from build123d import *

# Parameters (mm, degrees)
F0_R          = 2.5
F1_DEPTH      = 1.5
F1_DEPTH_BACK = 1.5
F3_DEPTH      = 2
F2_R          = 5.7
F2_R_2        = 4.2
F4_DEPTH      = 10


with BuildPart() as f1:
    # F0 (on Right) → F1 (new body, two sides)
    with BuildSketch(Plane.YZ) as f1_sk:
        with BuildLine():
            ThreePointArc((-5.5, 0), (0, -5.5), (5.5, 0))
            ThreePointArc((5.5, 0), (0, 5.5), (-5.5, 0))
        make_face()
        Circle(F0_R, mode=Mode.SUBTRACT)
        with BuildLine():
            Line((5.5, -6), (5.5, 0))
            ThreePointArc((5.5, 0), (0, -5.5), (-5.5, 0))
            Line((-5.5, 0), (-5.5, -6))
            Line((-5.5, -6), (5.5, -6))
        make_face()
    extrude(amount=F1_DEPTH)
    extrude(f1_sk.sketch, amount=-F1_DEPTH_BACK)

    # F2 (on face) → F3 (join)
    with BuildSketch(Plane(origin=(0, 0, -6), x_dir=(1, 0, 0), z_dir=(0, 0, -1))):
        with BuildLine():
            ThreePointArc((1.5, -3.9230090492), (3.4597687784, -2.38117618), (4.2, 0))
            ThreePointArc((4.2, 0), (3.4597687784, 2.38117618), (1.5, 3.9230090492))
            Line((1.5, 3.9230090492), (1.5, -3.9230090492))
        make_face()
        with BuildLine():
            Line((1.5, -3.9230090492), (1.5, 3.9230090492))
            ThreePointArc((1.5, 3.9230090492), (0, 4.2), (-1.5, 3.9230090492))
            Line((-1.5, 3.9230090492), (-1.5, -3.9230090492))
            ThreePointArc((-1.5, -3.9230090492), (0, -4.2), (1.5, -3.9230090492))
        make_face()
        with BuildLine():
            Line((-1.5, -3.9230090492), (-1.5, 3.9230090492))
            ThreePointArc((-1.5, 3.9230090492), (-4.2, 0), (-1.5, -3.9230090492))
        make_face()
    extrude(amount=F3_DEPTH)

    # F2 (on face) → F4 (join)
    with BuildSketch(Plane(origin=(0, 0, -6), x_dir=(1, 0, 0), z_dir=(0, 0, -1))):
        Circle(F2_R)
        Circle(F2_R_2, mode=Mode.SUBTRACT)
    extrude(amount=F4_DEPTH)


solid = f1.part
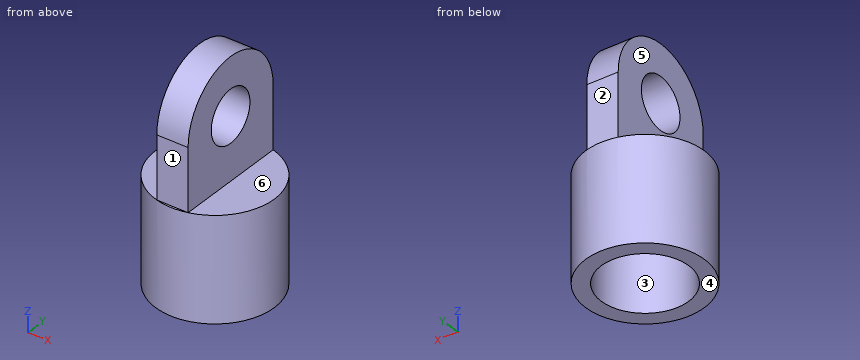
Work out the finished part from the listing and answer in its coordinate system (mm). Face numbers are marked on the shaded views. A direction names the side the tool comes from. Round coordinates to 2 decimals unless told otherwise and drop trailing zeros. Loops run counter-clockwise (first coordinate to the right, second up) from the corner with the lowest first, then second, coordinate; pieces in that order, holes last. Notation, with made-up numbers: (33.5, 49) -> (90.5, 49) arc R16 ccw to (90.5, 57) -> close; hole circle Ø9 at (23, 72). An arc over 180 degrees is marked (long way). Use one line per item in the form item = value.
(1) Find section B-B on y = 0. Give the vertices of the cut face in (x, z), then the cut area to 3 significant figures.
Answer list:
outline = (-5.7, -16) -> (-4.2, -16) -> (-4.2, -8) -> (4.2, -8) -> (4.2, -16) -> (5.7, -16) -> (5.7, -6) -> (1.5, -6) -> (1.5, -2.5) -> (-1.5, -2.5) -> (-1.5, -6) -> (-5.7, -6) -> close; (-1.5, 2.5) -> (1.5, 2.5) -> (1.5, 5.5) -> (-1.5, 5.5) -> close
area = 66.3 mm2
(2) Find section A-A on x = 0. Give the vertices of the cut face in (y, z), then the cut area to 3 significant figures.
Answer list:
outline = (-5.7, -16) -> (-4.2, -16) -> (-4.2, -8) -> (4.2, -8) -> (4.2, -16) -> (5.7, -16) -> (5.7, -6) -> (5.5, -6) -> (5.5, 0) arc R5.5 ccw to (-5.5, 0) -> (-5.5, -6) -> (-5.7, -6) -> close; hole circle Ø5 at (0, 0)
area = 141 mm2
(3) Flat-ended cylindrical pins translate along their axes: P1, Ø3.5, axis at x = -4, y = -2, coming from the +Z side; P2, Ø5, axis at y = 4, z = -6, coming from the -X side; P3, Ø5, axis at x = -2, y = -3.5, coming from the +Z side. Find the tip coordinate at first contact, or state that the pin passes through.
Answer list:
P1 = -6
P2 = -5.5
P3 = 5.4
(4) Find section D-D on z = -3.5. Give the vertices of the cut face in (x, y), then the cut area to 3 significant figures.
Answer list:
outline = (-1.5, -5.5) -> (1.5, -5.5) -> (1.5, 5.5) -> (-1.5, 5.5) -> close
area = 33.0 mm2
(5) Find section C-C on y = 5.25. Give the vertices of the cut face in (x, z), then the cut area to 3 significant figures.
Answer list:
outline = (-2.22, -16) -> (2.22, -16) -> (2.22, -6) -> (1.5, -6) -> (1.5, 1.64) -> (-1.5, 1.64) -> (-1.5, -6) -> (-2.22, -6) -> close
area = 67.3 mm2
(6) A tool of negligible diameter and unlimited length cuts with its end or side. For the marked faces 4, 5 and 6, from which of +Z, -Z, +X, -X, +Y, -Y can it reach the whole face along a straight path? Write none if from no direction.
Answer list:
face_4 = -Z, +X, -X, +Y, -Y
face_5 = +Z, -X, +Y, -Y
face_6 = +Z, +X, +Y, -Y
(7) For a pull along Y with two mould halves and no side action, classify the marked faces 1, 2 and 3 as released by +Y, released by -Y, zero draft, split by the parting line, or undercut.
Answer list:
face_1 = released by -Y
face_2 = released by +Y
face_3 = undercut
(8) Straight lines are drawn through the part: line 1 (Y direction, x = 0, z = -11.75); line 2 (Z direction, x = 0.55, y = 0). For each, find the intervals that lie inside material, in ascending order.
Answer list:
line_1 = -5.7 to -4.2, 4.2 to 5.7
line_2 = -8 to -2.5, 2.5 to 5.5
